Autodesk Inventor part; units mm, degrees
ref_plane "YZ Plane" through (0, 0, 0) normal (1, 0, 0) x (0, 1, 0)
ref_plane "XZ Plane" through (0, 0, 0) normal (0, 1, 0) x (-1, 0, 0)
ref_plane "XY Plane" through (0, 0, 0) normal (0, 0, 1) x (1, 0, 0)
sketch "Sketch1" plane through (0, 0, 0) normal (1, 0, 0) x (0, 1, 0)
  line L0 (0, 0) -> (7, 0)
  line L1 (7.5, -50) -> (7, -50)
  line L2 (7, -50) -> (7, -51.1)
  line L3 (7, -51.1) -> (7.5, -51.1)
  line L4 (7.5, -51.1) -> (7.5, -58.1)
  line L5 (7.5, -58.1) -> (10, -58.1)
  line L6 (10, -58.1) -> (10, -80.8)
  line L7 (10, -80.8) -> (9.5, -80.8)
  line L8 (9.5, -80.8) -> (9.5, -82.1)
  line L9 (9.5, -82.1) -> (10, -82.1)
  line L10 (10, -82.1) -> (10, -502.1)
  line L11 (10, -502.1) -> (9.5, -502.1)
  line L12 (9.5, -502.1) -> (9.5, -503.4)
  line L13 (9.5, -503.4) -> (10, -503.4)
  line L14 (10, -503.4) -> (10, -526.1)
  line L15 (10, -526.1) -> (7.5, -526.1)
  line L16 (7.5, -526.1) -> (7.5, -533.1)
  line L17 (7.5, -533.1) -> (7, -533.1)
  line L18 (7, -533.1) -> (7, -534.2)
  line L19 (7, -534.2) -> (7.5, -534.2)
  line L20 (7.5, -534.2) -> (7.5, -573.1)
  line L21 (7.5, -573.1) -> (0, -573.1)
  line L22 (0, -573.1) -> (0, 0)
  line L23 (6, -573.1) -> (6, -582.9) construction
  line L24 (6, -582.9) -> (0, -582.9)
  line L25 (0, -582.9) -> (0, -573.1)
  line L26 (6, -580.1) -> (5.5, -580.1)
  line L27 (5.5, -580.1) -> (5.5, -581.2)
  line L28 (5.5, -581.2) -> (6, -581.2)
  line L29 (6, -582.9) -> (6, -581.2)
  line L30 (6, -580.1) -> (6, -573.1)
  line L31 (7.5, -50) -> (7.5, -45)
  line L32 (7.5, -45) -> (7, -45)
  line L33 (7, -45) -> (7, 0)
  line L34 (0, 0) -> (7, 0)
  point P0 (8.75, -526.1)
  point P1 (9.75, -82.1)
  point P2 (9.75, -502.1)
  point P3 (7.5, -47.5)
  point P4 (7, -50.55)
  dimension "d15" = 50
  dimension "d16" = 1.1
  dimension "d17" = 7
  dimension "d18" = 10
  dimension "d19" = 0.5
  dimension "d20" = 1.3
  dimension "d21" = 1.3
  dimension "d22" = 7.5
  dimension "d23" = 0.5
  dimension "d24" = 1.1
  dimension "d25" = 7
  dimension "d26" = 468
  dimension "d27" = 47
  dimension "d28" = 420
  dimension "d29" = 24
  dimension "d32" = 6
  dimension "d33" = 0.5
  dimension "d34" = 7
  dimension "d35" = 1.1
  dimension "d36" = 1.7
  dimension "d52" = 5
  dimension "d53" = 7
  dimension "d54" = 7.5
  dimension "d55" = 7
  dimension "d56" = 7.5
revolve "Revolution1" add sketch "Sketch1" angle 360 about axis through (0, 0, -573.1) along (0, 0, 1)
sketch "Sketch2" plane through (0, 0, -580.1) normal (0, 0, -1) x (-1, 0, 0)
  circle A0 centre (0, 0) radius 6
  circle A1 centre (0, 0) radius 6
  line L0 (0, 6) -> (2, 6)
  line L1 (2, 6) -> (2, 4)
  line L2 (2, 4) -> (-2, 4)
  line L3 (-2, 4) -> (-2, 6)
  line L4 (-2, 6) -> (0, 6)
  dimension "d37" = 2
  dimension "d38" = 2
  dimension "d39" = 4
extrude "Extrusion1" cut sketch "Sketch2" against normal blind 7 contours L1 L2 L3 A0 | A0 L0 L1 | L3 L4 A0 picked at (0, 4.6667)
sketch "Sketch3" plane through (0, 0, -502.1) normal (0, 0, -1) x (-1, 0, 0)
  circle A0 centre (0, 0) radius 10
  line L0 (0, 10) -> (-2, 10)
  line L1 (-2, 10) -> (-2, 8)
  line L2 (-2, 8) -> (2, 8)
  line L3 (2, 8) -> (2, 10)
  line L4 (2, 10) -> (0, 10)
  point P0 (2, 9.798)
  point P1 (-2, 9.798)
  dimension "d42" = 2
  dimension "d43" = 2
  dimension "d44" = 4
extrude "Extrusion2" cut sketch "Sketch3" against normal blind 7 contours L3 L2 L1 A0 picked at (0, 8.6667)
sketch "Sketch4" plane through (0, 0, -82.1) normal (0, 0, 1) x (1, 0, 0)
  circle A0 centre (0, 0) radius 10
  line L0 (0, 10) -> (-2, 10)
  line L1 (-2, 8) -> (-2, 9.2871)
  line L2 (-2, 10) -> (-2, 8)
  line L3 (2, 8) -> (-2, 8)
  line L4 (-2, 8) -> (2, 8)
  line L5 (2, 8) -> (2, 10)
  line L6 (2, 10) -> (0, 10)
  point P0 (0, 0)
  point P1 (-2, 9.2871)
  dimension "d47" = 2
  dimension "d48" = 2
  dimension "d49" = 4
extrude "Extrusion3" cut sketch "Sketch4" against normal blind 7 contours L5 L3 L1 L2 A0 | A0 L6 L5 | L2 L0 A0 picked at (0, 8.6667)
properties part number "P201" material "Steel, Mild"
Model file for the job. Use its own axes, mm. A direction names the side the tool comes from. Round coordinates to 2 decimals unless told otherwise and drop trailing zeros. Write each loop counter-clockwise with the first axis right and the second up, starting at its lowest first coordinate (ties: lowest second). Pieces come first, ordered by that corner, then holes. Notation, with made-up numbers: (-7, -23) -> (2, -23) arc R26 ccw to (2, 8) -> close; hole circle Ø1 at (-16.75, 37.25). An arc over 180 degrees is marked (long way). Answer as CSV lines item,"result".
1. Slice it at A-A, the plane z = -142. List the corners of the cut face in (x, y).
Resolved:
outline,"circle Ø20 at (0, 0)"
2. Pin check, flat tips, straight feed: pin 1 Ø0.6 at (x, y) = (0, 9) entering from -Z; pin 2 Ø1.2 at (x, y) = (-0.5, 9) entering from +Z; pin 3 Ø1.5 at (y, z) = (-0.5, -392.5) entering from -X; pin 4 Ø4.5 at (x, z) = (0.5, -500) entering from +Y. Stop position of each tip, or through.
Resolved:
pin 1,"z = -526.1"
pin 2,"z = -58.1"
pin 3,"x = -10"
pin 4,"y = 9.8"
3. Mould opens along Z. For faces 1 (the face through (-7, 4, -58.1)), 2 (the face through (-8.43, 4.38, -81.46)), 3 (the face through (-9.76, -2.17, -295.04)) say: +Z half, -Z half, draft (parallel to the pull), parting line (faces both ways), or undercut.
Resolved:
face 1,"+Z half"
face 2,"undercut"
face 3,"draft"
4. Tool access for faces 4 (the face through (-0.33, -7.493, -47.465)), 5 (the face through (0, 0, -582.9)), 6 (the face through (0, -6, -577)), 7 (the face through (-2.681, 6.466, -533.658)): list every direction of +Z, -Z, +X, -X, +Y, -Y with a clear straight run to the whole face (end or side of a thin tool).
Resolved:
face 4,"+Z"
face 5,"-Z, +X, -X, +Y, -Y"
face 6,"-Z"
face 7,"none"
5. Drill centre lines: line 1 (Z direction, x = 7, y = -1); line 2 (X direction, y = 7.25, z = -524.5); line 3 (X direction, y = 8, z = -235.5). Where is each one in solid material? Low to high.
Resolved:
line 1,"-573.1 to -534.2, -533.1 to -51.1, -50 to -45"
line 2,"-6.89 to 6.89"
line 3,"-6 to 6"
